```python
from build123d import *

# Parameters (mm, degrees)
SKETCH1_W           = 10.2
SKETCH1_H           = 16
BOSS_EXTRUDE1_DEPTH = 5.8
SKETCH2_R           = 1.5
CUT_EXTRUDE1_DEPTH  = 3
FILLET1_R           = 2


with BuildPart() as part:
    # Sketch1 → Boss-Extrude1 (new body)
    with BuildSketch(Plane.XY):
        with BuildLine():
            Line((-15, 25), (-15, 20))
            Line((-15, 20), (15, 20))
            Line((15, 20), (15, 25))
            Line((15, 25), (17, 25))
            Line((17, 25), (17, 19))
            ThreePointArc((17, 19), (16.707106781, 18.292893219), (16, 18))
            Line((16, 18), (12.1, 18))
            ThreePointArc((12.1, 18), (8.564466094, 16.535533906), (7.1, 13))
            Line((7.1, 13), (7.1, 4))
            ThreePointArc((7.1, 4), (7.685786438, 2.585786438), (9.1, 2))
            Line((9.1, 2), (14.9, 2))
            Line((14.9, 2), (14.9, 0))
            Line((14.9, 0), (-14.9, 0))
            Line((-14.9, 0), (-14.9, 2))
            Line((-14.9, 2), (-9.1, 2))
            ThreePointArc((-9.1, 2), (-7.685786438, 2.585786438), (-7.1, 4))
            Line((-7.1, 4), (-7.1, 13))
            ThreePointArc((-7.1, 13), (-8.564466094, 16.535533906), (-12.1, 18))
            Line((-12.1, 18), (-16, 18))
            ThreePointArc((-16, 18), (-16.707106781, 18.292893219), (-17, 19))
            Line((-17, 19), (-17, 25))
            Line((-17, 25), (-15, 25))
        make_face()
        with Locations((0, 10)):
            Rectangle(SKETCH1_W, SKETCH1_H, mode=Mode.SUBTRACT)
    extrude(amount=BOSS_EXTRUDE1_DEPTH)

    # Sketch2 → Cut-Extrude1 (cut, through all)
    with BuildSketch(Plane(origin=(0, 2, 0), x_dir=(1, 0, 0), z_dir=(0, 1, 0))):
        with Locations((-12, -2.9)):
            Circle(SKETCH2_R)
        with Locations((12, -2.9)):
            Circle(SKETCH2_R)
    extrude(amount=-CUT_EXTRUDE1_DEPTH, mode=Mode.SUBTRACT)

    # Fillet1
    fillet1_edges = [part.edges().sort_by_distance(p)[0] for p in [
        (-5.1, 18, 2.9),
        (-5.1, 2, 2.9),
        (5.1, 2, 2.9),
        (5.1, 18, 2.9),
    ]]
    fillet(fillet1_edges, radius=FILLET1_R)


solid = part.part
```
Model file for the job. Use its own axes, mm. A direction names the side the tool comes from. Coordinates: 2 decimals unless noted, no trailing zeros. Loops run counter-clockwise (first coordinate to the right, second up) from the corner with the lowest first, then second, coordinate; pieces in that order, holes last. Notation, with made-up numbers: (18, 29.25) - (27, 29.25) arc R25 cw to (27, 67.25) - close; hole circle Ø11 at (-7.75, -34). An arc over 180 degrees is marked (long way). Write item = value, one per line. Start each with the question number.
Item 1: Pull direction X, two halves, no side cores. Call faces 6 (the face through (7.67, 2.6, 2.86)), 7 (the face through (-16.699, 18.285, 2.859)), 8 (the face through (-13.5, 1.01, 2.83)): +X half, -X half, draft (parallel to the pull), parting line (faces both ways), or undercut.
Item 2: 3-axis set-ups, long thin cutter, end or side, ignore diameter. For faces 1 (the face through (-7.1, 8, 3)), 2 (the face through (10.5, 1.01, 2.83)), 3 (the face through (0, 18, 3)), 4 (the face through (-15, 23, 3)), 5 (the face through (7.1, 9, 3)): which of +Z, -Z, +X, -X, +Y, -Y reach the whole face in a straight line?
Item 3: Drop flat-ended pins along their axis: pin 1 Ø1 at (y, z) = (1, 2) entering from -X; pin 2 Ø1 at (y, z) = (3.5, 1) entering from -X; pin 3 Ø2.5 at (x, z) = (12, 2.9) entering from +Y. Give the stop position or say it passes through.
Item 4: Saw through at A-A, the plane x = 2.5. List the corners of the cut face in (y, z).
Item 5: Wall check: probe 1 along X at (y, z) = (0.6, 2.9); probe 2 along Y at (x, z) = (0, 3.45); probe 3 along X at (y, z) = (10, 2.85). Give the ranges that are in metal, low to high. Write a range as [from, to].
Item 6: Saw through at D-D, the plane x = -12.5. List the corners of the cut face in (y, z), then the cut area to 3 significant figures.
Item 7: Saw through at C-C, the plane y = 8.75. List the corners of the cut face in (x, z).
Answers:
q1.face_6 = +X half
q1.face_7 = -X half
q1.face_8 = undercut
q2.face_1 = +Z, -Z, -X
q2.face_2 = -Y
q2.face_3 = +Z, -Z
q2.face_4 = +Z, -Z, +Y
q2.face_5 = +Z, -Z, +X
q3.pin_1 = -14.9
q3.pin_2 = -7.37
q3.pin_3 = 20
q4.outline = (0, 0) - (2, 0) - (2, 5.8) - (0, 5.8) - close; (18, 0) - (20, 0) - (20, 5.8) - (18, 5.8) - close
q5.probe_1 = [-14.9, -13.5], [-10.5, 10.5], [13.5, 14.9]
q5.probe_2 = [0, 2], [18, 20]
q5.probe_3 = [-7.1, -5.1], [5.1, 7.1]
q6.outline = (0, 0) - (2, 0) - (2, 1.49) - (0, 1.49) - close; (0, 4.31) - (2, 4.31) - (2, 5.8) - (0, 5.8) - close; (18, 0) - (20, 0) - (20, 5.8) - (18, 5.8) - close
q6.area = 17.5 mm2
q7.outline = (-7.1, 0) - (-5.1, 0) - (-5.1, 5.8) - (-7.1, 5.8) - close; (5.1, 0) - (7.1, 0) - (7.1, 5.8) - (5.1, 5.8) - close
